Design review of the part shown in the three views and the two pictorial views. Dimensions are in mm from the part's minimum x, y and z. Round coordinates to 2 decimals unless told otherwise and drop trailing zeros. Loops run counter-clockwise (first coordinate to the right, second up) from the corner with the lowest first, then second, coordinate; pieces in that order, holes last. Notation, with made-up numbers: M -18.75,58.5 L 29.25,58.5 A19 ccw 29.25,81.5 Z; hole C 62.5,78 d1. An arc over 180 degrees is marked long. Answer in a Markdown table with one row per item. Add a question column.
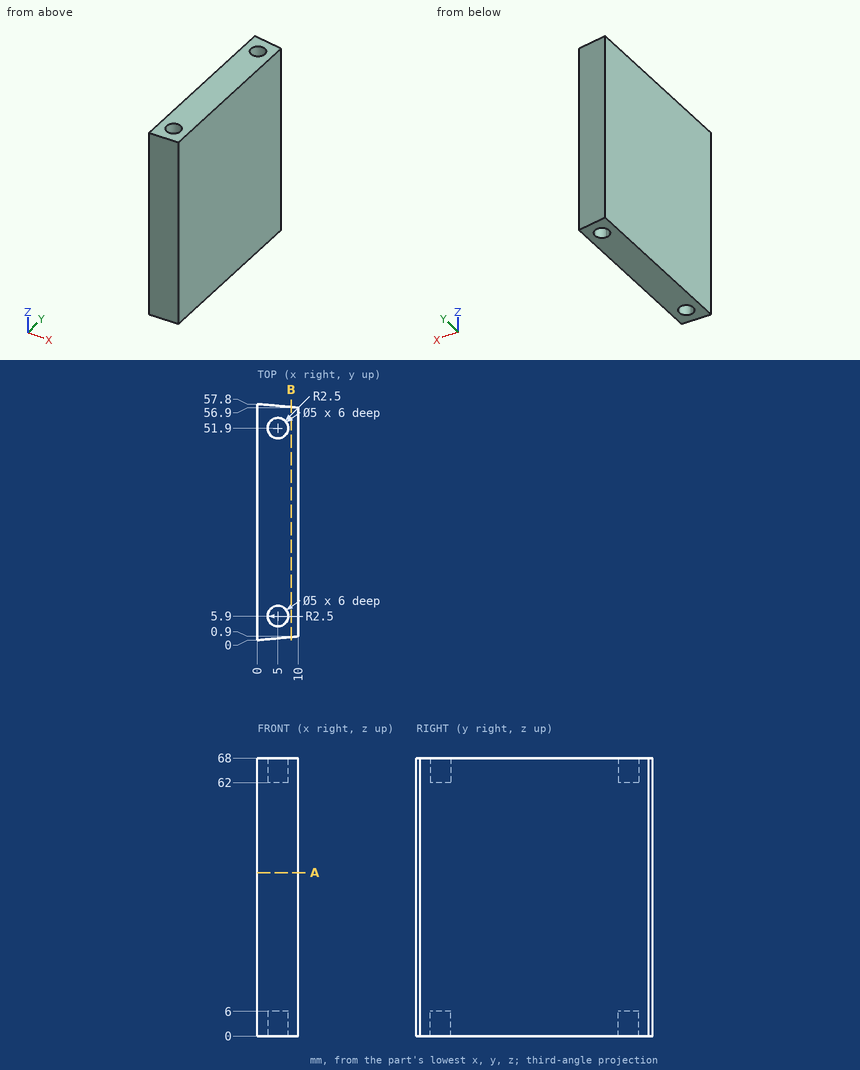
1. Take a section at A-A, the plane z = 40. State the section outline as (x, y) points, and give its area (3 significant figures).
2. Take a section at B-B, the plane x = 8.25. State the section outline as (y, z) points, and give its area (3 significant figures).
3. To check wall thickness, follow probe 1 along Y at (x, z) = (5, 65.35); probe 2 along X at (y, z) = (51, 65); probe 3 along Y at (x, z) = (7, 10.5). State the ranges of each line that lie inside material, in increasing order.
4. For pin 1 Ø2.5 at (x, y) = (6, 52.5) entering from -Z; pin 2 Ø1 at (x, z) = (7, 43.5) entering from -Y (3 decimals), all flat-tipped, find the tip position at first contact; note any pin that passes through.
Check sheet entries:
| question | item | result |
|---|---|---|
| 1 | outline | M 0,0 L 10,0.9 L 10,56.9 L 0,57.8 Z |
| 1 | area | 569 mm^2 |
| 2 | outline | M 0.74,0 L 57.06,0 L 57.06,68 L 0.74,68 Z |
| 2 | area | 3,830 mm^2 |
| 3 | probe 1 | y = 0.45 to 3.4, 8.4 to 49.4, 54.4 to 57.35 |
| 3 | probe 2 | x = 0 to 2.67, 7.33 to 10 |
| 3 | probe 3 | y = 0.63 to 57.17 |
| 4 | pin 1 | stops at z = 6 |
| 4 | pin 2 | stops at y = 0.585 |
